```python
from build123d import *

# Parameters (mm, degrees)
F1_W = 19.812
F1_H = 7.112
F0_W = 2.794
F0_H = 6.604


with BuildPart() as f2:
    # F1 (on Front) + F0 (on Front) → F2 (revolve)
    with BuildSketch(Plane.XZ):
        with Locations((9.906, 0)):
            Rectangle(F1_W, F1_H)
    with BuildSketch(Plane.XZ):
        with Locations((15.2908, 6.858)):
            Rectangle(F0_W, F0_H)
    revolve(axis=Axis((0, 0, 0), (0, 0, -1)))


solid = f2.part
```
Input: part model. Units: mm. Frame: model coordinates. A direction names the side the tool comes from. Round coordinates to 2 decimals unless told otherwise and drop trailing zeros. Loops run counter-clockwise (first coordinate to the right, second up) from the corner with the lowest first, then second, coordinate; pieces in that order, holes last.
1) Set-up query: faces 1 (the cylindrical face through (-2.579, -19.643, 0.05)), 2 (the flat face through (9, 15, 3.556)). Return all of +Z, -Z, +X, -X, +Y, -Y with unobstructed straight access to the full face (end or side cutting, diameter ignored); none if empty.
Ans:
face 1: +Z, -Z
face 2: +Z
2) Section query B-B on x = 0. Return the cut outline in (y, z), plus the area to 3 significant figures.
Ans:
outline: (-19.81, -3.56) - (19.81, -3.56) - (19.81, 3.56) - (16.69, 3.56) - (16.69, 10.16) - (13.89, 10.16) - (13.89, 3.56) - (-13.89, 3.56) - (-13.89, 10.16) - (-16.69, 10.16) - (-16.69, 3.56) - (-19.81, 3.56) - close
area: 319 mm2
3) Pull-direction query (Y, two-part tool) for faces 3 (the flat face through (4, -14, 10.16)), 4 (the cylindrical face through (-3.62, 16.29, 6.9)), 5 (the flat face through (0, 0, 3.556)); classes: released by +Y, released by -Y, zero draft, split by the parting line, or undercut.
Ans:
face 3: zero draft
face 4: split by the parting line
face 5: undercut
4) Pin query (flat end, axial travel): pin 1 (3 mm diameter, centred on x = 7, y = -7, fed in from +Z); pin 2 (2 mm diameter, centred on y = -8, z = -0.5, fed in from +X); pin 3 (2 mm diameter, centred on y = 10.5, z = 1, fed in from +X). Return the tip coordinate at first contact, or that it passes through.
Ans:
pin 1: stops at z = 3.56
pin 2: stops at x = 18.53
pin 3: stops at x = 17.39
5) Material intervals for line 1 (Y direction, x = 0, z = 6.25); line 2 (Z direction, x = -4, y = 8), sorted ascending.
Ans:
line 1: y = -16.69 to -13.89, 13.89 to 16.69
line 2: z = -3.56 to 3.56
6) Section query A-A on z = 7.5. Return the cut outline in (x, y).
Ans:
outline: circle Ø33.38 at (0, 0); hole circle Ø27.79 at (0, 0)
7) Section query D-D on z = 0.75. Return the cut outline in (x, y), plus the area to 3 significant figures.
Ans:
outline: circle Ø39.62 at (0, 0)
area: 1,230 mm2
